Check sheet for the modelled part. Datum: model origin and axes. Units: mm. Face numbers are marked on the shaded views. A direction names the side the tool comes from. Round coordinates to 2 decimals unless told otherwise and drop trailing zeros. Order: outer loops, then holes, each group sorted by start corner. A loop starts at its lowest first (then second) coordinate and runs counter-clockwise, first axis right, second up. Notation, with made-up numbers: M 10,53 L 14,53 A21 cw 14,73 Z; hole C -13,29.25 d9. An arc over 180 degrees is marked long. One line per item, written item: value. Start each with the question number.
(1) Cross-section at A-A, the plane z = -5. Enter the section's corners in (x, y).
(2) Cross-section at B-B, the plane x = -1. Enter the section's corners in (y, z).
(3) Access from +Z, -Z, +X, -X, +Y, -Y to the whole of each face (thin tool, end or side, straight path). Record for the marked faces 5 and 6.
(4) Cross-section at C-C, the plane y = 1.25. Enter the section's corners in (x, z).
(5) Thickness scan on L1, parallel to X at y = 0, z = 2.5; L2, parallel to X at y = 0, z = -3.25. Record the ranges inside material, lowest first.
(6) Release check for a two-part mould opening along Y. For the marked faces 1, 2, 3 and 4 record: released by +Y, released by -Y, zero draft, split by the parting line, or undercut.
(7) Cross-section at D-D, the plane x = 11.5. Enter the section's corners in (y, z).
(8) Depth check by flat-ended pin: pin 1 Ø1.9 at (y, z) = (-2, -2.5) entering from -X; pin 2 Ø7.5 at (x, y) = (0, 0) entering from +Z; pin 3 Ø2 at (y, z) = (-7, -3.5) entering from +X. Enter the tip coordinate at first touch or a pass-through.
from build123d import *

# Parameters (mm, degrees)
F0_R     = 12.7
F0_R_2   = 6.35
F1_DEPTH = 6.35
F2_W     = 38.1
F2_H     = 25.4
F3_DEPTH = 6.35
F5_DEPTH = 6.351


with BuildPart() as f1:
    # F0 (on Top) → F1 (new body, symmetric)
    with BuildSketch(Plane.XY):
        Circle(F0_R)
        Circle(F0_R_2, mode=Mode.SUBTRACT)
    extrude(amount=F1_DEPTH, both=True)

    # F2 (on Top) → F3 (join)
    with BuildSketch(Plane.XY):
        with Locations((19.05, 0)):
            Rectangle(F2_W, F2_H)
    extrude(amount=-F3_DEPTH)

    # F4 (on face) → F5 (cut, through all)
    with BuildSketch(Plane.XY):
        Polygon((38.1, -12.7), (38.1, 0), (25.4, -12.7), align=None)
    extrude(amount=-F5_DEPTH, mode=Mode.SUBTRACT)


solid = f1.part
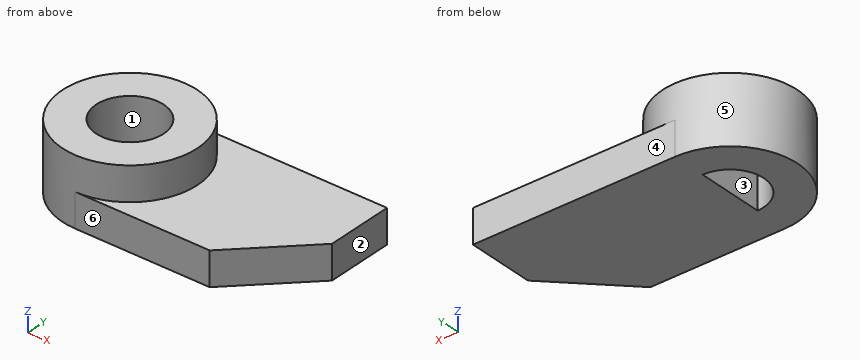
Values found:
1. outline: M 0,-12.7 L 25.4,-12.7 L 38.1,0 L 38.1,12.7 L 0,12.7 A12.7 ccw Z; hole M 0,-6.35 L 0,6.35 A6.35 ccw Z
2. outline: M -12.66,-6.35 L -6.27,-6.35 L -6.27,6.35 L -12.66,6.35 Z; M 6.27,-6.35 L 12.66,-6.35 L 12.66,6.35 L 6.27,6.35 Z
3. face 5: +Z
3. face 6: +Z, -Z, +X, -X, -Y
4. outline: M -12.64,-6.35 L -6.23,-6.35 L -6.23,6.35 L -12.64,6.35 Z; M 0,-6.35 L 38.1,-6.35 L 38.1,0 L 12.64,0 L 12.64,6.35 L 6.23,6.35 L 6.23,0 L 0,0 Z
5. L1: -12.7 to -6.35, 6.35 to 12.7
5. L2: -12.7 to -6.35, 0 to 38.1
6. face 1: undercut
6. face 2: zero draft
6. face 3: undercut
6. face 4: released by +Y
7. outline: M -12.7,-6.35 L 12.7,-6.35 L 12.7,0 L 5.39,0 L 5.39,6.35 L -5.39,6.35 L -5.39,0 L -12.7,0 Z
8. pin 1: x = -12.66
8. pin 2: z = 0
8. pin 3: x = 32.1
